Work out the finished part from the listing and answer in its coordinate system (mm). Face numbers are marked on the shaded views. A direction names the side the tool comes from. Round coordinates to 2 decimals unless told otherwise and drop trailing zeros. Loops run counter-clockwise (first coordinate to the right, second up) from the corner with the lowest first, then second, coordinate; pieces in that order, holes last.
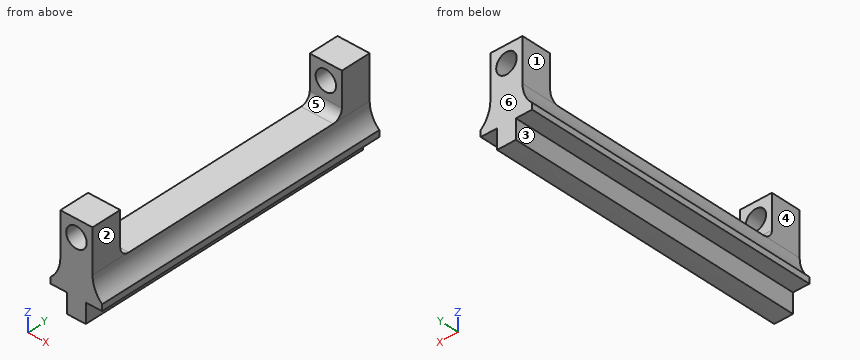
```python
from build123d import *

# Parameters (mm, degrees)
BOSS_EXTRUDE1_DEPTH   = 50.8
CUT_EXTRUDE1_DEPTH    = 99.34985718
SKETCH2_W             = 5.436248728
SKETCH2_H             = 7.283946563
BOSS_EXTRUDE2_DEPTH   = 5.08
FILLET1_R             = 1.5875
FILLET1_OF_MIRROR1_R  = 1.5875
F_4_CLEARANCE_HOLE1_D = 3.4544


with BuildPart() as part:
    # Sketch1 → Boss-Extrude1 (new body)
    with BuildSketch(Plane(origin=(0, 0, 0), x_dir=(1, 0, 0), z_dir=(0, 1, 0))):
        with BuildLine():
            Line((-2.718124364, 75.815452903), (2.718124364, 75.815452903))
            ThreePointArc((2.718124364, 75.815452903), (4.340809806, 79.470419596), (8.140147873, 80.718185524))
            Line((8.140147873, 80.718185524), (8.140147873, 83.423799917))
            ThreePointArc((8.140147873, 83.423799917), (0, 83.82), (-8.140147873, 83.423799917))
            Line((-8.140147873, 83.423799917), (-8.140147873, 80.718185524))
            ThreePointArc((-8.140147873, 80.718185524), (-4.340809806, 79.470419596), (-2.718124364, 75.815452903))
        make_face()
    extrude(amount=-BOSS_EXTRUDE1_DEPTH)

    # Sketch3 → Cut-Extrude1 (cut, through all)
    with BuildSketch(Plane(origin=(0, 0, 0), x_dir=(1, 0, 0), z_dir=(0, 1, 0))):
        Polygon((37.412226228, 86.104380481), (-3.175, 86.104380481), (-9.73961955, 86.104380481), (-9.73961955, 76.768037091), (-4.340809806, 76.768037091), (-4.340809806, 80.528090721), (-1.5875, 80.528090721), (-1.5875, 83.82), (0, 83.82), (40.587226228, 83.82), (87.99570433, 149.711789591), (84.82070433, 151.996170072), align=None)
    cut_extrude1 = extrude(amount=-CUT_EXTRUDE1_DEPTH, mode=Mode.SUBTRACT)

    # Mirror2: Cut-Extrude1 across plane
    add(cut_extrude1.mirror(Plane(origin=(0, 0, 0), x_dir=(0, 0, 1), z_dir=(1, 0, 0))), mode=Mode.SUBTRACT)

    # Sketch2 → Boss-Extrude2 (add)
    with BuildSketch(Plane(origin=(0, 0, 0), x_dir=(1, 0, 0), z_dir=(0, 1, 0))):
        with Locations((0, 72.173479622)):
            Rectangle(SKETCH2_W, SKETCH2_H)
    boss_extrude2 = extrude(amount=-BOSS_EXTRUDE2_DEPTH)

    # Fillet1
    fillet1_edges = [part.edges().sort_by_distance(p)[0] for p in [
        (0, -5.08, -75.815452903),
    ]]
    fillet(fillet1_edges, radius=FILLET1_R)

    # Mirror1: Boss-Extrude2 across plane
    add(boss_extrude2.mirror(Plane(origin=(0, -25.4, 0), x_dir=(0, 0, 1), z_dir=(0, -1, 0))))

    # Fillet1 of Mirror1
    fillet1_of_mirror1_edges = [part.edges().sort_by_distance(p)[0] for p in [
        (0, -45.72, -75.815452903),
    ]]
    fillet(fillet1_of_mirror1_edges, radius=FILLET1_OF_MIRROR1_R)

    # #4 Clearance Hole1 (through all)
    with Locations(Plane(origin=(0, 0, 0), x_dir=(1, 0, 0), z_dir=(0, 1, 0))):
        with Locations((0, 71.379729622)):
            Hole(F_4_CLEARANCE_HOLE1_D / 2)


solid = part.part
```
1. Which of the six approach directions +Z, -Z, +X, -X, +Y, -Y give full straight-line access (tool end or side, diameter ignored) to the marked faces 1, 2 and 3?
Answer key:
face 1: +Z, -X, +Y, -Y
face 2: +Z, +X, +Y, -Y
face 3: -Z, -X, +Y, -Y
2. Determine the mould class of the marked faces 4, 5 and 6 for opening direction Y: +Y half, -Y half, draft (parallel to the pull), parting line (faces both ways), or undercut.
Answer key:
face 4: draft
face 5: undercut
face 6: +Y half
3. Consider probe 1 along Z at (x, y) = (0, -4.05); probe 2 along Z at (x, y) = (0.5, -30); probe 3 along X at (y, z) = (-31.5, -76). Determine where each line is inside the solid, lowest interval first.
Answer key:
probe 1: z = -83.82 to -73.11, -69.65 to -68.53
probe 2: z = -83.82 to -75.82
probe 3: x = -2.72 to 2.72
4. Find section C-C (x = 3.25). Write down the section's boundary in (y, z).
Answer key:
outline: (-50.8, -80.53) - (0, -80.53) - (0, -78.04) - (-50.8, -78.04) - close
5. Find section A-A (x = 0). Write down the section's boundary in (y, z) (1 decimal), then the cut area to 3 significant figures.
Answer key:
outline: (-50.8, -83.8) - (0, -83.8) - (0, -73.1) - (-5.1, -73.1) - (-5.1, -74.2) arc R1.6 cw to (-6.7, -75.8) - (-44.1, -75.8) arc R1.6 cw to (-45.7, -74.2) - (-45.7, -73.1) - (-50.8, -73.1) - close; (-50.8, -69.7) - (-45.7, -69.7) - (-45.7, -68.5) - (-50.8, -68.5) - close; (-5.1, -69.7) - (0, -69.7) - (0, -68.5) - (-5.1, -68.5) - close
area: 447 mm2
6. Given pin 1 (2 mm diameter, centred on y = -48, z = -70.5, fed in from +X); pin 2 (2 mm diameter, centred on x = -3, y = -34.5, fed in from -Z); pin 3 (4.5 mm diameter, centred on x = -1, z = -71.5, fed in from -Y); pin 4 (3 mm diameter, centred on x = 2.5, y = -18, fed in from -Z), each flat-ended and moving along its own axis, determine where each tip first touches the part or whether it passes through.
Answer key:
pin 1: stops at x = 2.72
pin 2: stops at z = -80.53
pin 3: stops at y = -50.8
pin 4: stops at z = -83.81
7. Find section B-B (y = -11.5). Write down the section's boundary in (x, z).
Answer key:
outline: (-4.34, -80.53) - (-1.59, -80.53) - (-1.59, -83.8) arc R83.82 ccw to (1.59, -83.8) - (1.59, -80.53) - (4.34, -80.53) - (4.34, -79.47) arc R4.93 cw to (2.72, -75.82) - (-2.72, -75.82) arc R4.93 cw to (-4.34, -79.47) - close
